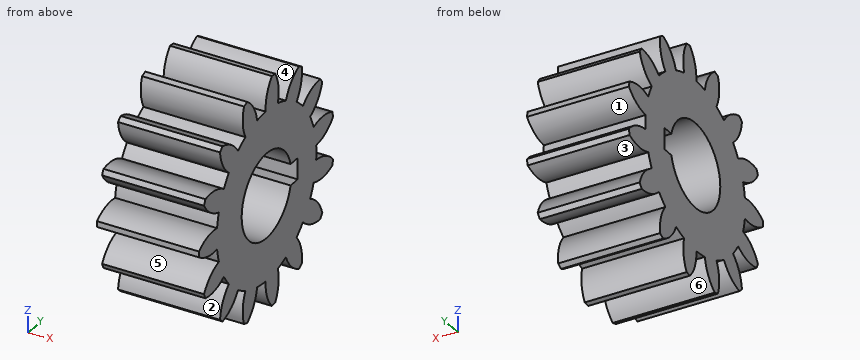
```python
from build123d import *

# Parameters (mm, degrees)
SPUR_START             = -48.028721504
SPUR_GEAR_AI_OUTLINE_R = 3.96875
SPUR_GEAR_AI_DEPTH     = 9.525
CUT_EXTRUDE1_DEPTH     = 38.391363975


# Read off the part's stored shape, not the designer's step: spur gear_ai
with BuildPart() as part:
    # spur gear_ai outline → spur gear_ai (new body)
    with BuildSketch(Plane.YZ.offset(SPUR_START)):
        with BuildLine():
            ThreePointArc((14.065180693, 15.046177845), (14.228771479, 15.265443857), (14.386753515, 15.488784863))
            ThreePointArc((14.386753515, 15.488784863), (13.653794557, 16.82563811), (12.455383467, 17.768090388))
            ThreePointArc((12.455383467, 17.768090388), (12.758302122, 18.376947995), (13.008079359, 19.009465686))
            ThreePointArc((13.008079359, 19.009465686), (14.510351432, 18.74949635), (15.994272276, 19.099331116))
            ThreePointArc((15.994272276, 19.099331116), (16.054536374, 19.366178952), (16.108019174, 19.634468198))
            ThreePointArc((16.108019174, 19.634468198), (14.894680646, 20.557623143), (13.416547762, 20.931158437))
            ThreePointArc((13.416547762, 20.931158437), (13.445633024, 21.610585655), (13.416547762, 22.290012873))
            ThreePointArc((13.416547762, 22.290012873), (14.894680646, 22.663548167), (16.108019174, 23.586703112))
            ThreePointArc((16.108019174, 23.586703112), (16.054536374, 23.854992358), (15.994272276, 24.121840194))
            ThreePointArc((15.994272276, 24.121840194), (14.510351432, 24.47167496), (13.008079359, 24.211705624))
            ThreePointArc((13.008079359, 24.211705624), (12.758302122, 24.844223315), (12.455383467, 25.453080922))
            ThreePointArc((12.455383467, 25.453080922), (13.653794557, 26.3955332), (14.386753515, 27.732386447))
            ThreePointArc((14.386753515, 27.732386447), (14.228771479, 27.955727454), (14.065180693, 28.174993465))
            ThreePointArc((14.065180693, 28.174993465), (12.567260927, 27.891018444), (11.300606153, 27.042495538))
            ThreePointArc((11.300606153, 27.042495538), (10.815155171, 27.518735647), (10.290780511, 27.951746631))
            ThreePointArc((10.290780511, 27.951746631), (11.002253642, 29.300157333), (11.128097767, 30.81955481))
            ThreePointArc((11.128097767, 30.81955481), (10.892933024, 30.959329889), (10.654301883, 31.093100991))
            ThreePointArc((10.654301883, 31.093100991), (9.401387132, 30.224418043), (8.589365776, 28.934058886))
            ThreePointArc((8.589365776, 28.934058886), (7.952179933, 29.171675171), (7.29701841, 29.353968))
            ThreePointArc((7.29701841, 29.353968), (7.398533415, 30.875184664), (6.895503115, 32.314408745))
            ThreePointArc((6.895503115, 32.314408745), (6.623817785, 32.346449516), (6.351407781, 32.371595469))
            ThreePointArc((6.351407781, 32.371595469), (5.560138388, 31.068407768), (5.343156318, 29.559327181))
            ThreePointArc((5.343156318, 29.559327181), (4.664410836, 29.517233628), (3.991745829, 29.417288215))
            ThreePointArc((3.991745829, 29.417288215), (3.465749841, 30.848278661), (2.420823624, 31.958474427))
            ThreePointArc((2.420823624, 31.958474427), (2.15959457, 31.877240748), (1.900507868, 31.789413589))
            ThreePointArc((1.900507868, 31.789413589), (1.707701498, 30.277054127), (2.123276886, 28.810185853))
            ThreePointArc((2.123276886, 28.810185853), (1.520333024, 28.49566082), (0.946474424, 28.130758636))
            ThreePointArc((0.946474424, 28.130758636), (-0.116083071, 29.224091616), (-1.522227969, 29.813296133))
            ThreePointArc((-1.522227969, 29.813296133), (-1.727831871, 29.632834046), (-1.928796828, 29.447219888))
            ThreePointArc((-1.928796828, 29.447219888), (-1.4898022, 27.987189356), (-0.513526115, 26.816168245))
            ThreePointArc((-0.513526115, 26.816168245), (-0.936413884, 26.283595967), (-1.312240712, 25.716831914))
            ThreePointArc((-1.312240712, 25.716831914), (-2.727633872, 26.283460223), (-4.251862224, 26.249794677))
            ThreePointArc((-4.251862224, 26.249794677), (-4.366290191, 26.001307717), (-4.474384734, 25.750000935))
            ThreePointArc((-4.474384734, 25.750000935), (-3.479495269, 24.594751875), (-2.11132549, 23.922058116))
            ThreePointArc((-2.11132549, 23.922058116), (-2.281036031, 23.263525179), (-2.393847214, 22.59289791))
            ThreePointArc((-2.393847214, 22.59289791), (-3.917341702, 22.534846366), (-5.296100578, 21.884131836))
            ThreePointArc((-5.296100578, 21.884131836), (-5.299566976, 21.610585655), (-5.296100578, 21.337039474))
            ThreePointArc((-5.296100578, 21.337039474), (-3.917341702, 20.686324945), (-2.393847214, 20.6282734))
            ThreePointArc((-2.393847214, 20.6282734), (-2.281036031, 19.957646131), (-2.11132549, 19.299113194))
            ThreePointArc((-2.11132549, 19.299113194), (-3.479495269, 18.626419435), (-4.474384734, 17.471170375))
            ThreePointArc((-4.474384734, 17.471170375), (-4.366290191, 17.219863593), (-4.251862224, 16.971376633))
            ThreePointArc((-4.251862224, 16.971376633), (-2.727633872, 16.937711087), (-1.312240712, 17.504339396))
            ThreePointArc((-1.312240712, 17.504339396), (-0.936413884, 16.937575343), (-0.513526115, 16.405003065))
            ThreePointArc((-0.513526115, 16.405003065), (-1.4898022, 15.233981954), (-1.928796828, 13.773951422))
            ThreePointArc((-1.928796828, 13.773951422), (-1.727831871, 13.588337264), (-1.522227969, 13.407875177))
            ThreePointArc((-1.522227969, 13.407875177), (-0.116083071, 13.997079694), (0.946474424, 15.090412674))
            ThreePointArc((0.946474424, 15.090412674), (1.520333024, 14.72551049), (2.123276886, 14.410985457))
            ThreePointArc((2.123276886, 14.410985457), (1.707701498, 12.944117183), (1.900507868, 11.431757721))
            ThreePointArc((1.900507868, 11.431757721), (2.15959457, 11.343930562), (2.420823624, 11.262696883))
            ThreePointArc((2.420823624, 11.262696883), (3.465749841, 12.372892649), (3.991745829, 13.803883095))
            ThreePointArc((3.991745829, 13.803883095), (4.664410836, 13.703937682), (5.343156318, 13.661844129))
            ThreePointArc((5.343156318, 13.661844129), (5.560138388, 12.152763542), (6.351407781, 10.849575841))
            ThreePointArc((6.351407781, 10.849575841), (6.623817785, 10.874721795), (6.895503115, 10.906762565))
            ThreePointArc((6.895503115, 10.906762565), (7.398533415, 12.345986646), (7.29701841, 13.86720331))
            ThreePointArc((7.29701841, 13.86720331), (7.952179933, 14.049496139), (8.589365776, 14.287112424))
            ThreePointArc((8.589365776, 14.287112424), (9.401387132, 12.996753267), (10.654301883, 12.128070319))
            ThreePointArc((10.654301883, 12.128070319), (10.892933024, 12.261841421), (11.128097767, 12.4016165))
            ThreePointArc((11.128097767, 12.4016165), (11.002253642, 13.921013977), (10.290780511, 15.269424679))
            ThreePointArc((10.290780511, 15.269424679), (10.815155171, 15.702435663), (11.300606153, 16.178675772))
            ThreePointArc((11.300606153, 16.178675772), (12.567260927, 15.330152866), (14.065180693, 15.046177845))
        make_face()
        with Locations((5.495433024, 21.610585655)):
            Circle(SPUR_GEAR_AI_OUTLINE_R, mode=Mode.SUBTRACT)
    extrude(amount=SPUR_GEAR_AI_DEPTH)

    # Sketch1 → Cut-Extrude1 (cut, through all)
    with BuildSketch(Plane(origin=(-38.503721504, 0, 0), x_dir=(0, 0, -1), z_dir=(1, 0, 0))):
        with BuildLine():
            Line((-20.610585655, 9.336133034), (-20.610585655, 10.464183024))
            Line((-20.610585655, 10.464183024), (-22.610585655, 10.464183024))
            Line((-22.610585655, 10.464183024), (-22.610585655, 9.336133034))
            ThreePointArc((-22.610585655, 9.336133034), (-21.610585655, 9.464183024), (-20.610585655, 9.336133034))
        make_face()
    extrude(amount=-CUT_EXTRUDE1_DEPTH, mode=Mode.SUBTRACT)


solid = part.part
```
Here's how the part is built. I have some questions about the finished solid (model axes, mm). Face numbers are marked on the shaded views. A direction names the side the tool comes from. Coordinates: 2 decimals unless noted, no trailing zeros. Write each loop counter-clockwise with the first axis right and the second up, starting at its lowest first coordinate (ties: lowest second). Pieces come first, ordered by that corner, then holes. Notation, with made-up numbers: M 83.5,-5.75 L 142.5,-5.75 A17 cw 142.5,21.25 Z; hole C -33,14 d10. An arc over 180 degrees is marked long. Answer as CSV lines item,"result". Start each with the question number.
Q1. I need wall thicknesses on probe 1 along Z at (x, y) = (-40, -1.25); probe 2 along Y at (x, z) = (-43.75, 31); probe 3 along Z at (x, y) = (-38.75, 14). Which ranges of each line are inside material? Lowest first, please. Write a range as [from, to].
Q2. Will these pins go through, and if not, where does the flat tip stop? pin 1 Ø1 at (x, y) = (-42, -0.5) entering from -Z; pin 2 Ø2 at (x, z) = (-46.5, 26.5) entering from +Y; pin 3 Ø1.5 at (y, z) = (2, 22) entering from -X; pin 4 Ø1 at (x, z) = (-42, 15.5) entering from -Y.
Q3. Suppose I cut it at B-B, the plane y = 7.75. List the corners of the cut face in (x, z) for me, then the cut area to 3 significant figures.
Q4. Suppose I cut it at A-A, the plane z = 24.75. List the corners of the cut face in (x, y) for me.
Q5. If we mould it in two halves opening along Y, with no side actions, what happens to the marked faces 1, 2 and 3? For each: pulls with the +Y half, pulls with the -Y half, needs draft (parallel to the pull), parting line crosses it, or undercut.
Q6. For the marked faces 4, 5 and 6, which set-ups out of +Z, -Z, +X, -X, +Y, -Y let a thin tool reach every point of the face, with its end or its side?
Entries:
1,probe 1,"z = [13.47, 15.62], [17.4, 25.82], [27.6, 29.75]"
1,probe 2,"y = [1.72, 3.37], [5.54, 7.38], [10.45, 10.82]"
1,probe 3,"z = [15.05, 16.35], [18.77, 20.86], [22.36, 24.45], [26.88, 28.18]"
2,pin 1,"stops at z = 13.55"
2,pin 2,"stops at y = 14.31"
2,pin 3,"stops at x = -48.03"
2,pin 4,"stops at y = -1.61"
3,outline,"M -48.03,13.99 L -38.5,13.99 L -38.5,18.34 L -48.03,18.34 Z; M -48.03,24.88 L -38.5,24.88 L -38.5,29.23 L -48.03,29.23 Z"
3,area,"83.0 mm²"
4,outline,"M -48.03,-3.67 L -38.5,-3.67 L -38.5,3.07 L -48.03,3.07 Z; M -48.03,7.92 L -38.5,7.92 L -38.5,12.8 L -48.03,12.8 Z"
5,face 1,"pulls with the +Y half"
5,face 2,"pulls with the -Y half"
5,face 3,"undercut"
6,face 4,"+Z, +X, -X"
6,face 5,"+X, -X, -Y"
6,face 6,"-Z, +X, -X"
